```python
from build123d import *
from OCP.BRepFilletAPI import BRepFilletAPI_MakeChamfer

# Parameters (mm, degrees)
SKETCH_1_W           = 276
SKETCH_1_H           = 276
EXTRUDE_1_DEPTH      = 6
SKETCH_4_R           = 6.5
SKETCH_4_R_2         = 2
CUT_EXTRUDE_1_DEPTH  = 10
SKETCH_5_R           = 2.4
CUT_EXTRUDE_2_DEPTH  = 196.253681143
FILLET_1_R           = 90
EXTRUDE_1_2_DEPTH    = 5
CHAMFER_2_SIZE       = 1.2
CHAMFER_2_SIZE2      = 3.296972903
SKETCH_9_W           = 33
SKETCH_9_H           = 33
EXTRUDE_2_DEPTH      = 11
FILLET_2_R           = 1
FILLET_3_R           = 10
CHAMFER_5_SIZE       = 3
CHAMFER_5_SIZE2      = 5.196152423
SKETCH_6_R           = 103
CUT_EXTRUDE_3_DEPTH  = 10
CHAMFER_6_SIZE       = 2
SKETCH_13_R          = 4.5
CUT_EXTRUDE_6_DEPTH  = 196.47122551
SKETCH_18_W          = 352.666964083
SKETCH_18_H          = 12.846548741
SKETCH_18_W_2        = 47.896370642
SKETCH_18_H_2        = 198.133814491
CUT_EXTRUDE_10_DEPTH = 196.900484949
CHAMFER_7_SIZE       = 4.5
CHAMFER_8_SIZE       = 1
FILLET_4_R           = 120
FILLET_5_R           = 80


with BuildPart() as part:
    # Эскиз1 → Extrude 1 (new body)
    with BuildSketch(Plane(origin=(0, 0, 0), x_dir=(1, 0, 0), z_dir=(0, 1, 0))):
        Rectangle(SKETCH_1_W, SKETCH_1_H)
    extrude(amount=EXTRUDE_1_DEPTH)

    # Эскиз4 → Cut-Extrude 1 (cut)
    with BuildSketch(Plane(origin=(0, 6, 0), x_dir=(1, 0, 0), z_dir=(0, 1, 0))):
        with Locations(Location((66, 114, 0), (0, 0, 270))):
            Circle(SKETCH_4_R)
        with Locations(Location((-120, 0, 0), (0, 0, 270))):
            Circle(SKETCH_4_R_2)
        with Locations(Location((66, -114, 0), (0, 0, 90))):
            Circle(SKETCH_4_R)
    extrude(amount=-CUT_EXTRUDE_1_DEPTH, mode=Mode.SUBTRACT)

    # Эскиз5 → Вырез-Вытянуть2 (cut, through all)
    with BuildSketch(Plane(origin=(0, 6, 0), x_dir=(1, 0, 0), z_dir=(0, 1, 0))):
        with Locations(Location((-85, 85, 0), (0, 0, 270))):
            Circle(SKETCH_5_R)
        with Locations(Location((85, 85, 0), (0, 0, 270))):
            Circle(SKETCH_5_R)
        with Locations(Location((85, -85, 0), (0, 0, 270))):
            Circle(SKETCH_5_R)
        with Locations(Location((-85, -85, 0), (0, 0, 270))):
            Circle(SKETCH_5_R)
        with Locations(Location((-90, 0, 0), (0, 0, 270))):
            Circle(SKETCH_5_R)
        with Locations(Location((0, 90, 0), (0, 0, 270))):
            Circle(SKETCH_5_R)
        with Locations(Location((0, -90, 0), (0, 0, 90))):
            Circle(SKETCH_5_R)
        with Locations(Location((90, 0, 0), (0, 0, 90))):
            Circle(SKETCH_5_R)
    extrude(amount=-CUT_EXTRUDE_2_DEPTH, mode=Mode.SUBTRACT)

    # Скругление1
    fillet_1_edges = [part.edges().sort_by_distance(p)[0] for p in [
        (138, 3, 138),
        (-138, 3, 138),
        (-138, 3, -138),
        (138, 3, -138),
    ]]
    fillet(fillet_1_edges, radius=FILLET_1_R)

    # Extrude 1 2: read off the stored shape, not the designer's step
    # Extrude 1 2 outline → Extrude 1 2 (add)
    # profile 1 of 2: a face of its own
    with BuildSketch(Plane(origin=(0, 6, 0), x_dir=(1, 0, 0), z_dir=(0, 1, 0))):
        Polygon((79.8, -106.032566285), (66, -98.06513257), (52.2, -106.032566285), (52.2, -121.967433715), (66, -129.93486743), (79.8, -121.967433715), align=None)
        Polygon((57.2, -108.919317631), (66, -103.838635262), (74.8, -108.919317631), (74.8, -119.080682369), (66, -124.161364738), (57.2, -119.080682369), align=None, mode=Mode.SUBTRACT)
    # profile 2 of 2: a face of its own
    with BuildSketch(Plane(origin=(0, 6, 0), x_dir=(1, 0, 0), z_dir=(0, 1, 0))):
        Polygon((52.2, 121.967433715), (52.2, 106.032566285), (66, 98.06513257), (79.8, 106.032566285), (79.8, 121.967433715), (66, 129.93486743), align=None)
        Polygon((66, 103.838635262), (57.2, 108.919317631), (57.2, 119.080682369), (66, 124.161364738), (74.8, 119.080682369), (74.8, 108.919317631), align=None, mode=Mode.SUBTRACT)
    extrude(amount=EXTRUDE_1_2_DEPTH)

    # Фаска2: one chamfer whose edges measure the first distance from different faces: ONE call of the kernel's chamfer builder (chamfer() names one face for all edges)
    chamfer_2_edges_1 = [part.edges().sort_by_distance(p)[0] for p in [
        (70.4, 11, 106.378976446),
        (61.6, 11, 106.378976447),
        (57.2, 11, 114),
        (61.6, 11, 121.621023554),
        (70.4, 11, 121.621023553),
        (74.8, 11, 114),
    ]]
    chamfer_2_side_1 = [part.faces().sort_by_distance(p)[0] for p in [
        (72.689201518, 11, 102.413963108),
    ]]
    chamfer_2_edges_2 = [part.edges().sort_by_distance(p)[0] for p in [
        (74.8, 11, -114),
        (70.4, 11, -121.621023554),
        (61.6, 11, -121.621023553),
        (57.2, 11, -114),
        (61.6, 11, -106.378976446),
        (70.4, 11, -106.378976447),
    ]]
    chamfer_2_side_2 = [part.faces().sort_by_distance(p)[0] for p in [
        (52.621596964, 11, -114),
    ]]
    chamfer_2 = BRepFilletAPI_MakeChamfer(part.part.solid().wrapped)
    for e in chamfer_2_edges_1:
        chamfer_2.Add(CHAMFER_2_SIZE, CHAMFER_2_SIZE2, e.wrapped, chamfer_2_side_1[0].wrapped)  # the first distance lies on this face
    for e in chamfer_2_edges_2:
        chamfer_2.Add(CHAMFER_2_SIZE, CHAMFER_2_SIZE2, e.wrapped, chamfer_2_side_2[0].wrapped)  # the first distance lies on this face
    add(Compound.cast(chamfer_2.Shape()), mode=Mode.REPLACE)

    # Эскиз9 → Бобышка-Вытянуть2 (add)
    with BuildSketch(Plane(origin=(0, 6, 0), x_dir=(1, 0, 0), z_dir=(0, 1, 0))):
        with Locations((-120, 0)):
            Rectangle(SKETCH_9_W, SKETCH_9_H)
    extrude(amount=EXTRUDE_2_DEPTH)

    # Эскиз10 → Вырез-Повернуть1 (revolve, cut)
    with BuildSketch(Plane(origin=(0, 13, 0), x_dir=(1, 0, 0), z_dir=(0, 1, 0))):
        with BuildLine():
            Line((-131.5, 0), (-108.5, 0))
            ThreePointArc((-108.5, 0), (-120, 11.5), (-131.5, 0))
        make_face()
    revolve(axis=Axis((-131.5, 13, 0), (1, 0, 0)), mode=Mode.SUBTRACT)

    # Скругление2
    fillet_2_edges = [part.edges().sort_by_distance(p)[0] for p in [
        (-119.999999999, 1.675248347, -1.999999986),
        (-120, 17, -10.781929326),
    ]]
    fillet(fillet_2_edges, radius=FILLET_2_R)

    # Скругление3
    fillet_3_edges = [part.edges().sort_by_distance(p)[0] for p in [
        (-103.5, 11.5, 16.5),
        (-103.5, 11.5, -16.5),
        (-136.5, 11.5, -16.5),
        (-136.5, 11.5, 16.5),
    ]]
    fillet(fillet_3_edges, radius=FILLET_3_R)

    # Фаска5
    chamfer_5_edges = [part.edges().sort_by_distance(p)[0] for p in [
        (66, 0, 120.5),
        (66, 0, -120.5),
    ]]
    chamfer_5_side = [part.faces().sort_by_distance(p)[0] for p in [
        (-0.232742345, 0, 0),
    ]]
    chamfer(chamfer_5_edges, length=CHAMFER_5_SIZE, length2=CHAMFER_5_SIZE2, reference=chamfer_5_side[0])

    # Эскиз6 → Вырез-Вытянуть3 (cut)
    with BuildSketch(Plane(origin=(0, 6, 0), x_dir=(1, 0, 0), z_dir=(0, 1, 0))):
        with Locations(Location((0, 0, 0), (0, 0, 270))):
            Circle(SKETCH_6_R)
    extrude(amount=-CUT_EXTRUDE_3_DEPTH, mode=Mode.SUBTRACT)

    # Фаска6
    chamfer_6_edges = [part.edges().sort_by_distance(p)[0] for p in [
        (85, 6, -87.4),
        (85, 6, 82.6),
        (-85, 6, 82.6),
        (-85, 6, -87.4),
    ]]
    chamfer(chamfer_6_edges, length=CHAMFER_6_SIZE)

    # Эскиз13 → Вырез-Вытянуть6 (cut, through all)
    with BuildSketch(Plane(origin=(0, 6, 0), x_dir=(1, 0, 0), z_dir=(0, 1, 0))):
        with Locations(Location((126, 50, 0), (0, 0, 270))):
            Circle(SKETCH_13_R)
        with Locations(Location((126, -50, 0), (0, 0, 90))):
            Circle(SKETCH_13_R)
        with Locations(Location((106, -50, 0), (0, 0, 270))):
            Circle(SKETCH_13_R)
        with Locations(Location((106, 50, 0), (0, 0, 90))):
            Circle(SKETCH_13_R)
    extrude(amount=-CUT_EXTRUDE_6_DEPTH, mode=Mode.SUBTRACT)

    # Эскиз18 → Вырез-Вытянуть10 (cut, through all)
    with BuildSketch(Plane(origin=(0, 17, 0), x_dir=(1, 0, 0), z_dir=(0, 1, 0))):
        with Locations((-14.279105497, 137.42327437)):
            Rectangle(SKETCH_18_W, SKETCH_18_H)
        with Locations((-14.279105497, -137.42327437)):
            Rectangle(SKETCH_18_W, SKETCH_18_H)
        with Locations((156.948185321, -9.822497885)):
            Rectangle(SKETCH_18_W_2, SKETCH_18_H_2)
    extrude(amount=-CUT_EXTRUDE_10_DEPTH, mode=Mode.SUBTRACT)

    # Фаска7
    # the kernel refuses this chamfer: 4.5 mm, written as the material it takes off along each edge
    with BuildSketch(Plane(origin=(106, 6, -50), x_dir=(0, 0, -1), z_dir=(1, 0, 0))) as chamfer_7_piece_1:
        Polygon((4.5 + CHAMFER_7_SIZE, 0), (4.5, -CHAMFER_7_SIZE), (4.5, 0), align=None)
    revolve(axis=Axis((106, 6, -50), (0, 1, 0)), mode=Mode.SUBTRACT)
    with BuildSketch(Plane(origin=(106, 6, 50), x_dir=(0, 0, 1), z_dir=(-1, 0, 0))) as chamfer_7_piece_2:
        Polygon((4.5 + CHAMFER_7_SIZE, 0), (4.5, -CHAMFER_7_SIZE), (4.5, 0), align=None)
    revolve(axis=Axis((106, 6, 50), (0, 1, 0)), mode=Mode.SUBTRACT)
    with BuildSketch(Plane(origin=(126, 6, 50), x_dir=(0, 0, -1), z_dir=(1, 0, 0))) as chamfer_7_piece_3:
        Polygon((4.5 + CHAMFER_7_SIZE, 0), (4.5, -CHAMFER_7_SIZE), (4.5, 0), align=None)
    revolve(axis=Axis((126, 6, 50), (0, 1, 0)), mode=Mode.SUBTRACT)
    with BuildSketch(Plane(origin=(126, 6, -50), x_dir=(0, 0, 1), z_dir=(-1, 0, 0))) as chamfer_7_piece_4:
        Polygon((4.5 + CHAMFER_7_SIZE, 0), (4.5, -CHAMFER_7_SIZE), (4.5, 0), align=None)
    revolve(axis=Axis((126, 6, -50), (0, 1, 0)), mode=Mode.SUBTRACT)

    # Фаска8
    chamfer_8_edges = [part.edges().sort_by_distance(p)[0] for p in [
        (0, 0, -103),
        (113.584975562, 0, 109.632872564),
        (113.584975562, 0, -109.632872564),
        (-122.939803427, 0, 97.840002631),
        (0, 0, -131),
        (0, 0, 131),
        (133, 0, 0),
        (-138, 0, 0),
        (-122.939803427, 0, -97.840002631),
    ]]
    chamfer(chamfer_8_edges, length=CHAMFER_8_SIZE)

    # Скругление4
    # the kernel refuses this fillet: 120 mm, written as the material it takes off along each edge
    with BuildSketch(Plane(origin=(-82.799425283, -329.218710186, 131), x_dir=(1, 0, 0), z_dir=(0, 1, 0))) as fillet_4_piece_1:
        with BuildLine():
            CenterArc((64.799425283, 120), FILLET_4_R, 180, 90)
            Line((-55.200574717, 120), (-67.200574717, 120))
            ThreePointArc((-67.200574717, 120), (-67.200574717, 83), (-4.639923371, -11.066666667))
            Line((-4.639923371, -11.066666667), (0, -12))
            Line((0, -12), (64.799425283, -12))
            Line((64.799425283, -12), (64.799425283, 0))
        make_face()
    extrude(amount=665.437420372, mode=Mode.SUBTRACT)
    with BuildSketch(Plane(origin=(-82.799425283, -329.218710186, -131), x_dir=(1, 0, 0), z_dir=(0, 1, 0))) as fillet_4_piece_2:
        with BuildLine():
            CenterArc((64.799425283, -120), FILLET_4_R, 90, 90)
            Line((-55.200574717, -120), (-67.200574717, -120))
            ThreePointArc((-67.200574717, -120), (-67.200574717, -83), (-4.639923371, 11.066666667))
            Line((-4.639923371, 11.066666667), (0, 12))
            Line((0, 12), (64.799425283, 12))
            Line((64.799425283, 12), (64.799425283, 0))
        make_face()
    extrude(amount=665.437420372, mode=Mode.SUBTRACT)

    # Скругление5
    # the kernel refuses this fillet: 80 mm, written as the material it takes off along each edge
    with BuildSketch(Plane(origin=(82.799425283, -182.264690441, -131), x_dir=(-1, 0, 0), z_dir=(0, 1, 0))) as fillet_5_piece_1:
        with BuildLine():
            CenterArc((25.254593386, 80), FILLET_5_R, 199.405701267, 70.594298733)
            Line((-50.200574717, 53.419601085), (-51.709678079, 52.887993106))
            ThreePointArc((-51.709678079, 52.887993106), (-31.951505401, 20.271431924), (-0.618656449, -1.475555556))
            Line((-0.618656449, -1.475555556), (0, -1.6))
            Line((0, -1.6), (25.254593386, -1.6))
            Line((25.254593386, -1.6), (25.254593386, 0))
        make_face()
    extrude(amount=371.529380882, mode=Mode.SUBTRACT)
    with BuildSketch(Plane(origin=(82.799425283, -182.264690441, 131), x_dir=(-1, 0, 0), z_dir=(0, 1, 0))) as fillet_5_piece_2:
        with BuildLine():
            CenterArc((25.254593386, -80), FILLET_5_R, 90, 70.594298733)
            Line((-50.200574717, -53.419601085), (-51.709678079, -52.887993106))
            ThreePointArc((-51.709678079, -52.887993106), (-31.951505401, -20.271431924), (-0.618656449, 1.475555556))
            Line((-0.618656449, 1.475555556), (0, 1.6))
            Line((0, 1.6), (25.254593386, 1.6))
            Line((25.254593386, 1.6), (25.254593386, 0))
        make_face()
    extrude(amount=371.529380882, mode=Mode.SUBTRACT)


solid = part.part
```
Source: CAD feature listing. Evaluate the final solid. Frame: model axes, mm. A direction names the side the tool comes from. Give positions to 0.01 mm unless a question says otherwise; leave off trailing zeros. Put each result on its own line as item: value. Start each with the question number.
1) Cut plane A-A (x = 126). State how many separate pieces and enclosed holes the cut face has, then the cut area to 3 significant figures.
2) Reachability of faces 4 (the face through (-106.51, 11.58, -13.65)), 5 (the face through (59.2, 8.46, -126.01)), 6 (the face through (72.997, 8.465, 102.105)), 7 (the face through (72.8, 8.46, 126.01)) from +Z, -Z, +X, -X, +Y, -Y: full face, straight path, thin tool, end or side. Return the list, or none.
3) Contact query for flat-ended pins moving along their axis: P1, Ø5.5, axis at x = 69.5, z = -111, coming from the +Y side; P2, Ø5.5, axis at y = 11, z = 2, coming from the +X side; P3, Ø0.9, axis at y = 6.5, z = 115.5, coming from the -X side. Output: stop coordinate, or through.
4) Material intervals for probe 1 along X at (y, z) = (3.5, -52); probe 2 along X at (y, z) = (1.25, -52.5); probe 3 along X at (y, z) = (2.75, -30.5), sorted ascending.
5) Draft query along X for faces 1 (the face through (59.003, 8.465, 125.895)), 2 (the face through (-103.5, 11, 0)), 3 (the face through (82.76, 4.125, 86.165)). Return one class per face: released by +X, released by -X, zero draft, split by the parting line, or undercut.
Results are:
1. separate pieces: 3
1. enclosed holes: 0
1. area: 959 mm2
2. face 4: -Z, +X, +Y
2. face 5: -Z, -X, +Y
2. face 6: +X, +Y
2. face 7: +Z, +X, +Y
3. P1: stops at y = 6
3. P2: stops at x = -103.5
3. P3: stops at x = 52.2
4. probe 1: x = -130.78 to -88.91, 88.91 to 99.82, 112.18 to 119.82, 132.18 to 133
4. probe 2: x = -130.6 to -88.62, 88.62 to 102.26, 109.74 to 122.26, 129.74 to 133
4. probe 3: x = -136.41 to -98.38, 98.38 to 133
5. face 1: released by -X
5. face 2: released by +X
5. face 3: undercut
